The model under review builds one solid part; all positions refer to its coordinate system, in mm. Face numbers are marked on the shaded views. A direction names the side the tool comes from. Give positions to 0.01 mm unless a question says otherwise; leave off trailing zeros. Loops run counter-clockwise (first coordinate to the right, second up) from the corner with the lowest first, then second, coordinate; pieces in that order, holes last. Notation, with made-up numbers: M 7,36.25 L 63,36.25 A12 cw 63,51.25 Z; hole C -15,67.5 d3. An arc over 180 degrees is marked long. Write item = value, one per line. Start each with the question number.
1. We need section A-A on z = 0. Give the boundary of the cut face in (x, y).
2. Draft analysis for pull direction Z (two halves, no side actions). For the marked faces 1, 2 and 3, state which applies: pulls with the +Z half, pulls with the -Z half, needs draft (parallel to the pull), parting line crosses it, or undercut.
3. We need section B-B on x = 2.7. Give the boundary of the cut face in (y, z).
4. For the marked faces 4, 5 and 6, list the 3-axis set-ups (+Z, -Z, +X, -X, +Y, -Y) from which the entire face can be reached by the end or side of a thin tool; tool diameter is ignored.
5. For pin 1 (1.6 mm diameter, centred on x = 2, y = 8.5, fed in from -Z); pin 2 (1 mm diameter, centred on y = 6.45, z = 0, fed in from +X), all flat-tipped, find the tip position at first contact; note any pin that passes through.
6. We need section C-C on y = 10. Give the boundary of the cut face in (x, z).
7. Wall thickness on line 1 along Y through (x, z) = (2.2, 0); line 2 along Y through (x, z) = (1.2, 0); line 3 along X through (y, z) = (9.25, -6.5): over which ranges is each line inside the solid? List them lowest first. Write a range as from..to.
8. We need section D-D on y = 8.45. Give the boundary of the cut face in (x, z), then the cut area to 3 significant figures.
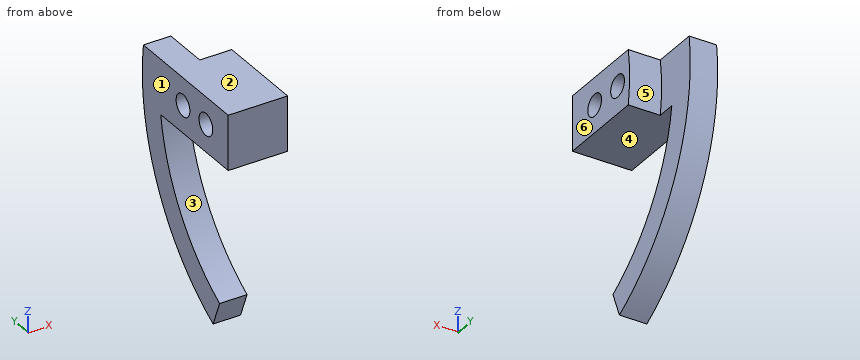
from build123d import *

# Parameters (mm, degrees)
CROQUIS1_R              = 0.6
SALIENTE_EXTRUIR1_DEPTH = 1.5
CROQUIS2_R              = 0.6
SALIENTE_EXTRUIR2_DEPTH = 1.75


with BuildPart() as part:
    # Croquis1 → Saliente-Extruir1 (new body)
    with BuildSketch(Plane(origin=(0, 0, 0), x_dir=(0, 0, -1), z_dir=(1, 0, 0))):
        with BuildLine():
            Line((-1.5, 4.5), (1.5, 4.5))
            Line((1.5, 4.5), (1.5, 10.392304845))
            ThreePointArc((1.5, 10.392304845), (5.887711766, 8.693954806), (9.09326674, 5.25))
            Line((9.09326674, 5.25), (10.495980844, 5.816733286))
            ThreePointArc((10.495980844, 5.816733286), (5.431514292, 10.700404315), (-1.5, 11.9058809))
            Line((-1.5, 11.9058809), (-1.5, 4.5))
        make_face()
        with Locations((0, 8.45)):
            Circle(CROQUIS1_R, mode=Mode.SUBTRACT)
        with Locations((0, 6.45)):
            Circle(CROQUIS1_R, mode=Mode.SUBTRACT)
    extrude(amount=SALIENTE_EXTRUIR1_DEPTH)

    # Croquis2 → Saliente-Extruir2 (add)
    with BuildSketch(Plane(origin=(1.5, 0, 0), x_dir=(0, 0, -1), z_dir=(1, 0, 0))):
        with BuildLine():
            Line((-1.5, 4.5), (1.5, 4.5))
            Line((1.5, 4.5), (1.5, 9.38083152))
            ThreePointArc((1.5, 9.38083152), (0, 9.5), (-1.5, 9.38083152))
            Line((-1.5, 9.38083152), (-1.5, 4.5))
        make_face()
        with Locations((0, 6.45)):
            Circle(CROQUIS2_R, mode=Mode.SUBTRACT)
        with Locations((0, 8.45)):
            Circle(CROQUIS2_R, mode=Mode.SUBTRACT)
    extrude(amount=SALIENTE_EXTRUIR2_DEPTH)


solid = part.part
Final values:
q1.outline = M 0,4.5 L 3.25,4.5 L 3.25,5.85 L 0,5.85 Z; M 0,7.05 L 3.25,7.05 L 3.25,7.85 L 0,7.85 Z; M 0,9.05 L 3.25,9.05 L 3.25,9.5 L 1.5,9.5 L 1.5,12 L 0,12 Z
q2.face_1 = needs draft
q2.face_2 = pulls with the +Z half
q2.face_3 = undercut
q3.outline = M 4.5,-1.5 L 9.38,-1.5 A9.5 ccw 9.38,1.5 L 4.5,1.5 Z; hole C 6.45,0 d1.2; hole C 8.45,0 d1.2
q4.face_4 = +X, -X, -Y
q4.face_5 = +X, +Y
q4.face_6 = +Z, -Z, +X, +Y, -Y
q5.pin_1 = -9.05
q5.pin_2 = through
q6.outline = M 0,-6.63 L 1.5,-6.63 L 1.5,-3.2 L 0,-3.2 Z; M 0,-1.5 L 1.5,-1.5 L 1.5,1.5 L 0,1.5 Z
q7.line_1 = 4.5..5.85, 7.05..7.85, 9.05..9.5
q7.line_2 = 4.5..5.85, 7.05..7.85, 9.05..12
q7.line_3 = 0..1.5
q8.outline = M 0,-8.52 L 1.5,-8.52 L 1.5,-6.23 L 0,-6.23 Z; M 0,-1.5 L 3.25,-1.5 L 3.25,-0.6 L 0,-0.6 Z; M 0,0.6 L 3.25,0.6 L 3.25,1.5 L 0,1.5 Z
q8.area = 9.28 mm²
